Can you work these out from the model? Positions are in its coordinate system, mm. Face numbers are marked on the shaded views. A direction names the side the tool comes from. Coordinates: 2 decimals unless noted, no trailing zeros. Order: outer loops, then holes, each group sorted by start corner. A loop starts at its lowest first (then second) coordinate and runs counter-clockwise, first axis right, second up. Notation, with made-up numbers: (-36, 88) -> (11, 88) arc R33 ccw to (11, 123) -> close; hole circle Ø5 at (57.5, 19). An arc over 180 degrees is marked (long way). Use a Markdown table: item, result. Add a question column.
1. For the marked faces 1 and 2, which set-ups out of +Z, -Z, +X, -X, +Y, -Y let a thin tool reach every point of the face, with its end or its side?
2. We'd pull the mould along X, two halves only. Please class the marked faces 3, 4, 5 and 6: pulls with the +X half, pulls with the -X half, needs draft (parallel to the pull), parting line crosses it, or undercut.
3. If I drill on line 1 along Z through (x, y) = (-19, 45); line 2 along Z through (x, y) = (0, 18); line 3 along X through (y, z) = (39, 0), over which ranges is the centre line in solid material (lowest first)? Write a range as from..to.
4. Suppose I cut it at A-A, the plane y = 26.5. List the corners of the cut face in (x, z) for me, then the cut area to 3 significant figures.
5. For pin 1 Ø1.2 at (x, z) = (1.5, 21.5) entering from -Y, with a flat end and sliding along its axis, tell me the tip position at first contact or that it passes through.
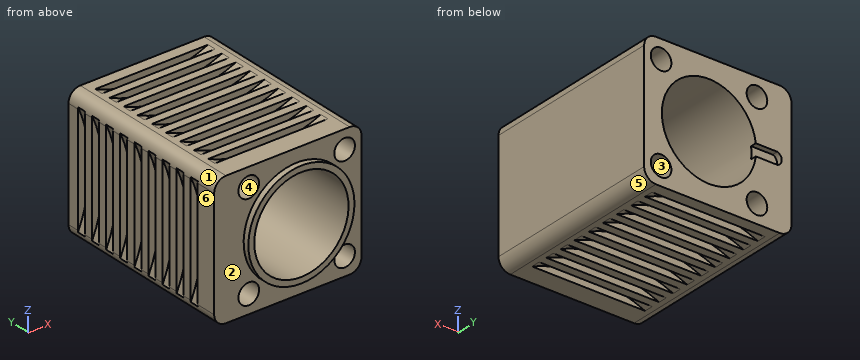
```python
from build123d import *

# Parameters (mm, degrees)
BOSS_EXTRUDE1_DEPTH     = 62
SKETCH2_R               = 18
BOSS_EXTRUDE2_DEPTH     = 2
SKETCH3_R               = 16
CUT_EXTRUDE1_DEPTH      = 74.391075752
CUT_EXTRUDE2_DEPTH      = 2
SKETCH5_R               = 3.5
CUT_EXTRUDE3_DEPTH      = 74.391075752
SKETCH6_W               = 48
SKETCH6_H               = 3
LPATTERN1_COUNT         = 9
LPATTERN1_PITCH         = 6
MIRROR1_COPY_1_SKETCH_W = 48
MIRROR1_COPY_1_SKETCH_H = 3
MIRROR1_COPY_2_SKETCH_W = 48
MIRROR1_COPY_2_SKETCH_H = 3
MIRROR1_COPY_3_SKETCH_W = 48
MIRROR1_COPY_3_SKETCH_H = 3
MIRROR1_COPY_4_SKETCH_W = 48
MIRROR1_COPY_4_SKETCH_H = 3
MIRROR1_COPY_5_SKETCH_W = 48
MIRROR1_COPY_5_SKETCH_H = 3
MIRROR1_COPY_6_SKETCH_W = 48
MIRROR1_COPY_6_SKETCH_H = 3
MIRROR1_COPY_7_SKETCH_W = 48
MIRROR1_COPY_7_SKETCH_H = 3
MIRROR1_COPY_8_SKETCH_W = 48
MIRROR1_COPY_8_SKETCH_H = 3
SKETCH10_W              = 48
SKETCH10_H              = 3
LPATTERN2_COUNT         = 9
LPATTERN2_PITCH         = 6


with BuildPart() as part:
    # Sketch1 → Boss-Extrude1 (new body)
    with BuildSketch(Plane(origin=(0, 0, 0), x_dir=(1, 0, 0), z_dir=(0, 1, 0))):
        with BuildLine():
            Line((-24, -22.5), (18, -22.5))
            ThreePointArc((18, -22.5), (20.828427125, -21.328427125), (22, -18.5))
            Line((22, -18.5), (22, 18.5))
            ThreePointArc((22, 18.5), (20.828427125, 21.328427125), (18, 22.5))
            Line((18, 22.5), (-24, 22.5))
            ThreePointArc((-24, 22.5), (-26.828427125, 21.328427125), (-28, 18.5))
            Line((-28, 18.5), (-28, -18.5))
            ThreePointArc((-28, -18.5), (-26.828427125, -21.328427125), (-24, -22.5))
        make_face()
    extrude(amount=BOSS_EXTRUDE1_DEPTH)

    # Sketch2 → Boss-Extrude2 (add)
    with BuildSketch(Plane.XZ):
        with Locations(Location((0, 0, 0), (0, 0, 270))):
            Circle(SKETCH2_R)
    extrude(amount=BOSS_EXTRUDE2_DEPTH)

    # Sketch3 → Cut-Extrude1 (cut, through all)
    with BuildSketch(Plane.XZ.offset(2)):
        with Locations(Location((0, 0, 0), (0, 0, 270))):
            Circle(SKETCH3_R)
    extrude(amount=-CUT_EXTRUDE1_DEPTH, mode=Mode.SUBTRACT)

    # Sketch4 → Cut-Extrude2 (cut)
    with BuildSketch(Plane(origin=(0, 62, 0), x_dir=(1, 0, 0), z_dir=(0, 1, 0))):
        with BuildLine():
            Line((-23.144533893, 2), (-8.5852446, 2))
            Line((-8.5852446, 2), (-8.5852446, -2))
            Line((-8.5852446, -2), (-23.144533893, -2))
            ThreePointArc((-23.144533893, -2), (-24.680199624, 0), (-23.144533893, 2))
        make_face()
    extrude(amount=-CUT_EXTRUDE2_DEPTH, mode=Mode.SUBTRACT)

    # Sketch5 → Cut-Extrude3 (cut, through all)
    with BuildSketch(Plane(origin=(0, 62, 0), x_dir=(1, 0, 0), z_dir=(0, 1, 0))):
        with Locations(Location((16.263455967, 16.263455967, 0), (0, 0, 270))):
            Circle(SKETCH5_R)
        with Locations(Location((16.263455967, -16.263455967, 0), (0, 0, 270))):
            Circle(SKETCH5_R)
        with Locations(Location((-16.263455967, -16.263455967, 0), (0, 0, 270))):
            Circle(SKETCH5_R)
        with Locations(Location((-16.263455967, 16.263455967, 0), (0, 0, 270))):
            Circle(SKETCH5_R)
    extrude(amount=-CUT_EXTRUDE3_DEPTH, mode=Mode.SUBTRACT)

    # Sketch6 → Cut-Revolve1 (revolve, cut)
    with BuildSketch(Plane(origin=(-3, 0, 0), x_dir=(0, 0, -1), z_dir=(1, 0, 0))):
        with Locations((-42.5, 56.5)):
            Rectangle(SKETCH6_W, SKETCH6_H)
    cut_revolve1 = revolve(axis=Axis((-3, 58, 66.5), (0, -1, 0)), mode=Mode.SUBTRACT)

    # LPattern1: Cut-Revolve1 ×9
    with Locations(*[(0, -i * LPATTERN1_PITCH, 0) for i in range(1, LPATTERN1_COUNT)]):
        add(cut_revolve1, mode=Mode.SUBTRACT)

    # Mirror1: Cut-Revolve1 across plane
    add(cut_revolve1.mirror(Plane.XY), mode=Mode.SUBTRACT)

    # Mirror1 copy 1 sketch → Mirror1 copy 1 (revolve, cut)
    with BuildSketch(Plane(origin=(-3, -6, 0), x_dir=(0, 0, 1), z_dir=(1, 0, 0))):
        with Locations((-42.5, -56.5)):
            Rectangle(MIRROR1_COPY_1_SKETCH_W, MIRROR1_COPY_1_SKETCH_H)
    revolve(axis=Axis((-3, 52, -66.5), (0, 1, 0)), mode=Mode.SUBTRACT)

    # Mirror1 copy 2 sketch → Mirror1 copy 2 (revolve, cut)
    with BuildSketch(Plane(origin=(-3, -12, 0), x_dir=(0, 0, 1), z_dir=(1, 0, 0))):
        with Locations((-42.5, -56.5)):
            Rectangle(MIRROR1_COPY_2_SKETCH_W, MIRROR1_COPY_2_SKETCH_H)
    revolve(axis=Axis((-3, 46, -66.5), (0, 1, 0)), mode=Mode.SUBTRACT)

    # Mirror1 copy 3 sketch → Mirror1 copy 3 (revolve, cut)
    with BuildSketch(Plane(origin=(-3, -18, 0), x_dir=(0, 0, 1), z_dir=(1, 0, 0))):
        with Locations((-42.5, -56.5)):
            Rectangle(MIRROR1_COPY_3_SKETCH_W, MIRROR1_COPY_3_SKETCH_H)
    revolve(axis=Axis((-3, 40, -66.5), (0, 1, 0)), mode=Mode.SUBTRACT)

    # Mirror1 copy 4 sketch → Mirror1 copy 4 (revolve, cut)
    with BuildSketch(Plane(origin=(-3, -24, 0), x_dir=(0, 0, 1), z_dir=(1, 0, 0))):
        with Locations((-42.5, -56.5)):
            Rectangle(MIRROR1_COPY_4_SKETCH_W, MIRROR1_COPY_4_SKETCH_H)
    revolve(axis=Axis((-3, 34, -66.5), (0, 1, 0)), mode=Mode.SUBTRACT)

    # Mirror1 copy 5 sketch → Mirror1 copy 5 (revolve, cut)
    with BuildSketch(Plane(origin=(-3, -30, 0), x_dir=(0, 0, 1), z_dir=(1, 0, 0))):
        with Locations((-42.5, -56.5)):
            Rectangle(MIRROR1_COPY_5_SKETCH_W, MIRROR1_COPY_5_SKETCH_H)
    revolve(axis=Axis((-3, 28, -66.5), (0, 1, 0)), mode=Mode.SUBTRACT)

    # Mirror1 copy 6 sketch → Mirror1 copy 6 (revolve, cut)
    with BuildSketch(Plane(origin=(-3, -36, 0), x_dir=(0, 0, 1), z_dir=(1, 0, 0))):
        with Locations((-42.5, -56.5)):
            Rectangle(MIRROR1_COPY_6_SKETCH_W, MIRROR1_COPY_6_SKETCH_H)
    revolve(axis=Axis((-3, 22, -66.5), (0, 1, 0)), mode=Mode.SUBTRACT)

    # Mirror1 copy 7 sketch → Mirror1 copy 7 (revolve, cut)
    with BuildSketch(Plane(origin=(-3, -42, 0), x_dir=(0, 0, 1), z_dir=(1, 0, 0))):
        with Locations((-42.5, -56.5)):
            Rectangle(MIRROR1_COPY_7_SKETCH_W, MIRROR1_COPY_7_SKETCH_H)
    revolve(axis=Axis((-3, 16, -66.5), (0, 1, 0)), mode=Mode.SUBTRACT)

    # Mirror1 copy 8 sketch → Mirror1 copy 8 (revolve, cut)
    with BuildSketch(Plane(origin=(-3, -48, 0), x_dir=(0, 0, 1), z_dir=(1, 0, 0))):
        with Locations((-42.5, -56.5)):
            Rectangle(MIRROR1_COPY_8_SKETCH_W, MIRROR1_COPY_8_SKETCH_H)
    revolve(axis=Axis((-3, 10, -66.5), (0, 1, 0)), mode=Mode.SUBTRACT)

    # Sketch10 → Cut-Revolve2 (revolve, cut)
    with BuildSketch(Plane.XY):
        with Locations((-48, 56.5)):
            Rectangle(SKETCH10_W, SKETCH10_H)
    cut_revolve2 = revolve(axis=Axis((-72, 58, 0), (0, -1, 0)), mode=Mode.SUBTRACT)

    # LPattern2: Cut-Revolve2 ×9
    with Locations(*[(0, -i * LPATTERN2_PITCH, 0) for i in range(1, LPATTERN2_COUNT)]):
        add(cut_revolve2, mode=Mode.SUBTRACT)


solid = part.part
```
Worked out:
| question | item | result |
|---|---|---|
| 1 | face 1 | +Z, -X, +Y, -Y |
| 1 | face 2 | -Y |
| 2 | face 3 | undercut |
| 2 | face 4 | undercut |
| 2 | face 5 | pulls with the +X half |
| 2 | face 6 | pulls with the -X half |
| 3 | line 1 | z = -21.25..-18.45, -14.08..14.08, 18.45..21.25 |
| 3 | line 2 | z = -22.5..-16, 16..22.5 |
| 3 | line 3 | x = -24..-16, 16..22 |
| 4 | outline | (-27.96, -19.08) arc R4 ccw to (-24, -22.5) -> (-22.18, -22.5) arc R48 cw to (16.18, -22.5) -> (18, -22.5) arc R4 ccw to (22, -18.5) -> (22, 18.5) arc R4 ccw to (18, 22.5) -> (16.18, 22.5) arc R48 cw to (-22.18, 22.5) -> (-24, 22.5) arc R4 ccw to (-27.96, 19.08) arc R48 cw to start; hole circle Ø7 at (-16.26, -16.26); hole circle Ø7 at (-16.26, 16.26); hole circle Ø32 at (0, 0); hole circle Ø7 at (16.26, -16.26); hole circle Ø7 at (16.26, 16.26) |
| 4 | area | 969 mm² |
| 5 | pin 1 | stops at y = 0 |
